Read the model definition and answer for the solid it produces. Units are mm, in the model's axes. Coordinates: 2 decimals unless noted, no trailing zeros. Write each loop counter-clockwise with the first axis right and the second up, starting at its lowest first coordinate (ties: lowest second). Pieces come first, ordered by that corner, then holes.
(1) Section B-B on x = -24 is taken. Write down the section's boundary in (y, z).
(2) The mould has two halves that part along Y. Classify faces 1 (the cylindrical face through (-2.15, -0.09, 1.97)), 2 (the conical face through (-77.65, 0.07, 0.17)), 3 (the flat face through (-37, 4, 2)): +Y half, -Y half, draft (parallel to the pull), parting line (faces both ways), or undercut.
(3) Section A-A on y = 0 is taken. Write down the section's boundary in (x, z), then the cut area to 3 significant figures.
(4) Find the intervals of material crossed by probe 1 along Y at (x, z) = (0, 2.3); probe 2 along X at (y, z) = (-0.25, 0.35); probe 3 along X at (y, z) = (-1.25, 2.05), in increasing order.
Autodesk Fusion 360 part; units mm, degrees
sketch "Sketch1" plane through (0, 0, 0) normal (0, 0, 1) x (1, 0, 0)
  circle A0 centre (0, 0) radius 2.15
  circle A1 centre (0, 0) radius 4
  circle A2 centre (-74.481, 0) radius 2.15
  circle A3 centre (-74.481, 0) radius 4
  line L0 (0, 4) -> (-74.481, 4)
  line L1 (-74.481, -4) -> (0, -4)
  dimension "d1" = 4.3
  dimension "d2" = 8
  dimension "d3" = 74.481
  dimension "d4" = 4.3
  dimension "d5" = 8
extrude "Extrude1" add sketch "Sketch1" along normal blind 4
chamfer "Chamfer1" distance 1 angle 45 8 edges at (-37.2405, -4, 4) (4, 0, 4) (-37.2405, 4, 4) (-78.481, 0, 4) (-78.481, 0, 0) (-37.2405, -4, 0) (4, 0, 0) (-37.2405, 4, 0)
Response:
1. outline: (-4, 1) - (-3, 0) - (3, 0) - (4, 1) - (4, 3) - (3, 4) - (-3, 4) - (-4, 3) - close
2. face 1: undercut
2. face 2: parting line
2. face 3: +Y half
3. outline: (-78.48, 1) - (-77.48, 0) - (-76.63, 0) - (-76.63, 4) - (-77.48, 4) - (-78.48, 3) - close; (-72.33, 0) - (-2.15, 0) - (-2.15, 4) - (-72.33, 4) - close; (2.15, 0) - (3, 0) - (4, 1) - (4, 3) - (3, 4) - (2.15, 4) - close
3. area: 294 mm2
4. probe 1: y = -4 to -2.15, 2.15 to 4
4. probe 2: x = -77.82 to -76.62, -72.35 to -2.14, 2.14 to 3.34
4. probe 3: x = -78.28 to -76.23, -72.73 to -1.75, 1.75 to 3.8
